Check sheet for the modelled part. Datum: model origin and axes. Units: mm. Face numbers are marked on the shaded views. A direction names the side the tool comes from. Coordinates: 2 decimals unless noted, no trailing zeros. Write each loop counter-clockwise with the first axis right and the second up, starting at its lowest first coordinate (ties: lowest second). Pieces come first, ordered by that corner, then holes. Notation, with made-up numbers: (-25, -17.75) -> (10, -17.75) arc R33 cw to (10, 17.25) -> close; hole circle Ø7 at (70.5, 23.25). An arc over 180 degrees is marked (long way). One line per item, written item: value. Start each with the question number.
1) Gauge pin test, flat ends, axial feed: P1, Ø3, axis at x = 7.5, z = 0, coming from the -Y side; P2, Ø2, axis at x = -7.5, z = 0, coming from the +Y side. Record the tip position at first contact, or that the pin passes through.
2) Sectioned sample at C-C on z = 8. Enter the section's corners in (x, y) (3 decimals).
3) Sectioned sample at B-B on y = -3.53. Enter the section's corners in (x, z) (3 decimals), plus the area to 3 significant figures.
4) Sectioned sample at A-A on x = -19. Enter the section's corners in (y, z) (3 decimals), plus the area to 3 significant figures.
5) Set-up check for the marked faces 1 and 2: record each of +Z, -Z, +X, -X, +Y, -Y from which the full face is reachable in a straight line by a thin tool's end or side.
6) Sectioned sample at D-D on x = 5.5. Enter the section's corners in (y, z), plus the area to 3 significant figures.
7) Scan lines: line 1 along X through (y, z) = (-14.5, 4.75) (3 decimals); line 2 along Y through (x, z) = (-4.5, 1.5). Record each from-to range of solid material in increasing order. Write a range as [from, to].
8) Draft check along X on the marked faces 3, 4 and 5. Enter one of: +X half, -X half, draft (parallel to the pull), parting line (faces both ways), or undercut.
```python
from build123d import *

# Parameters (mm, degrees)
BOSS_EXTRUDE1_DEPTH       = 12.5
M3X0_5_TAPPED_HOLE1_D     = 2.5
M3X0_5_TAPPED_HOLE1_DEPTH = 8
M3X0_5_TAPPED_HOLE1_TIP   = 0.751075774
F_2_5MM_DOWEL_HOLE1_D     = 2.5


with BuildPart() as part:
    # Sketch2 → Boss-Extrude1 (new body, symmetric)
    with BuildSketch(Plane.XY):
        Polygon((-23.075, -21), (-23.075, 9), (23.075, 9), (23.075, -21), (15, -21), (15, 0), (-15, 0), (-15, -21), align=None)
    extrude(amount=BOSS_EXTRUDE1_DEPTH, both=True)

    # M3x0.5 Tapped Hole1
    with Locations(Plane(origin=(0, 9, 0), x_dir=(1, 0, 0), z_dir=(0, 1, 0))):
        with Locations((-7.5, 0), (7.5, 0)):
            Hole(M3X0_5_TAPPED_HOLE1_D / 2, depth=M3X0_5_TAPPED_HOLE1_DEPTH)
            with Locations((0, 0, -(M3X0_5_TAPPED_HOLE1_DEPTH + M3X0_5_TAPPED_HOLE1_TIP / 2))):  # 118° drill point
                Cone(0, M3X0_5_TAPPED_HOLE1_D / 2, M3X0_5_TAPPED_HOLE1_TIP, mode=Mode.SUBTRACT)

    # Ø2.5mm Dowel Hole1 (through all)
    with Locations(Plane.ZY.offset(23.075)):
        with Locations((-9.795, -3.53), (9.795, -16.5), (-9.795, -16.5), (9.795, -3.53)):
            Hole(F_2_5MM_DOWEL_HOLE1_D / 2)


solid = part.part
```
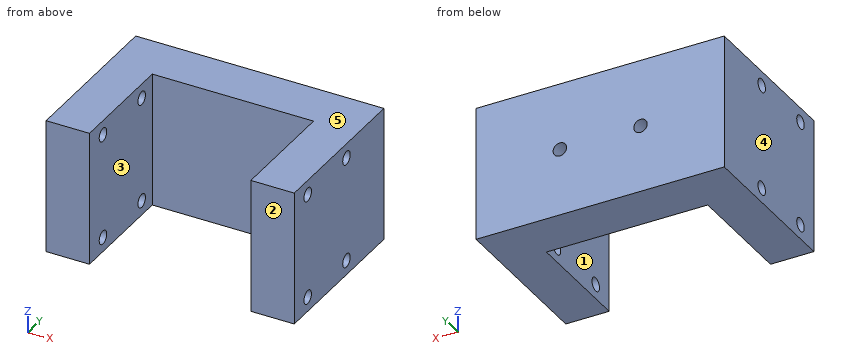
Answers:
1. P1: stops at y = 0
1. P2: stops at y = 0.85
2. outline: (-23.075, -21) -> (-15, -21) -> (-15, 0) -> (15, 0) -> (15, -21) -> (23.075, -21) -> (23.075, 9) -> (-23.075, 9) -> close
3. outline: (-23.075, -12.5) -> (-15, -12.5) -> (-15, -11.045) -> (-23.075, -11.045) -> close; (-23.075, -8.545) -> (-15, -8.545) -> (-15, 8.545) -> (-23.075, 8.545) -> close; (-23.075, 11.045) -> (-15, 11.045) -> (-15, 12.5) -> (-23.075, 12.5) -> close; (15, -12.5) -> (23.075, -12.5) -> (23.075, -11.045) -> (15, -11.045) -> close; (15, -8.545) -> (23.075, -8.545) -> (23.075, 8.545) -> (15, 8.545) -> close; (15, 11.045) -> (23.075, 11.045) -> (23.075, 12.5) -> (15, 12.5) -> close
3. area: 323 mm2
4. outline: (-21, -12.5) -> (9, -12.5) -> (9, 12.5) -> (-21, 12.5) -> close; hole circle Ø2.5 at (-16.5, -9.795); hole circle Ø2.5 at (-16.5, 9.795); hole circle Ø2.5 at (-3.53, -9.795); hole circle Ø2.5 at (-3.53, 9.795)
4. area: 730 mm2
5. face 1: +Z, -Z, -Y
5. face 2: +Z, -Z, +X, -X, -Y
6. outline: (0, -12.5) -> (9, -12.5) -> (9, 12.5) -> (0, 12.5) -> close
6. area: 225 mm2
7. line 1: x = [-23.075, -15], [15, 23.075]
7. line 2: y = [0, 9]
8. face 3: undercut
8. face 4: -X half
8. face 5: draft
